```python
from build123d import *

# Parameters (mm, degrees)
HOLE_WIZARD_M31_AT_2_COUNT = 2
HOLE_WIZARD_M31_AT_2_PITCH = 12
HOLE_WIZARD_M31_AT_3_COUNT = 2
HOLE_WIZARD_M31_AT_3_PITCH = 8.485281374
HOLE_WIZARD_M31_AT_4_COUNT = 2
HOLE_WIZARD_M31_AT_4_PITCH = 8.485281374


with BuildPart() as part:
    # Эскиз1 → Повернуть1 (revolve)
    with BuildSketch(Plane(origin=(0, 0, 0), x_dir=(0, 0, -1), z_dir=(1, 0, 0))):
        with BuildLine():
            Line((-4, 9), (-3, 9))
            Line((-3, 9), (-3, 9.539392014))
            ThreePointArc((-3, 9.539392014), (0, 10), (3, 9.539392014))
            Line((3, 9.539392014), (3, 0))
            Line((3, 0), (-4, 0))
            Line((-4, 0), (-4, 9))
        make_face()
    revolve(axis=Axis((0, 0, 0), (0, 0, 1)))

    # Эскиз2 → Цековка для винта с внутренним шестигранником M31 (revolve, cut)
    with BuildSketch(Plane(origin=(6, 0, -3), x_dir=(0, 1, 0), z_dir=(1, 0, 0))):
        Polygon((0, 0), (0, 7), (1.9, 7), (1.7, 6.8), (1.7, 3.6), (1.9, 3.4), (3, 3.4), (3, 0.25), (3.25, 0), align=None)
    hole_wizard_m31 = revolve(axis=Axis((6, 0, -9.35), (0, 0, 1)), mode=Mode.SUBTRACT)

    # Цековка для винта с внутренним шестигранником M31 at 2: Цековка для винта с внутренним шестигранником M31 ×2
    with Locations(*[(-i * HOLE_WIZARD_M31_AT_2_PITCH, 0, 0) for i in range(1, HOLE_WIZARD_M31_AT_2_COUNT)]):
        add(hole_wizard_m31, mode=Mode.SUBTRACT)

    # Цековка для винта с внутренним шестигранником M31 at 3: Цековка для винта с внутренним шестигранником M31 ×2
    with Locations(*[Vector(-0.707106781, 0.707106781, 0) * (i * HOLE_WIZARD_M31_AT_3_PITCH) for i in range(1, HOLE_WIZARD_M31_AT_3_COUNT)]):
        add(hole_wizard_m31, mode=Mode.SUBTRACT)

    # Цековка для винта с внутренним шестигранником M31 at 4: Цековка для винта с внутренним шестигранником M31 ×2
    with Locations(*[Vector(-0.707106781, -0.707106781, 0) * (i * HOLE_WIZARD_M31_AT_4_PITCH) for i in range(1, HOLE_WIZARD_M31_AT_4_COUNT)]):
        add(hole_wizard_m31, mode=Mode.SUBTRACT)


solid = part.part
```
The listing builds one solid part. Answer for the finished solid, in the listing's coordinates (mm). A direction names the side the tool comes from. Round coordinates to 2 decimals unless told otherwise and drop trailing zeros. Write each loop counter-clockwise with the first axis right and the second up, starting at its lowest first coordinate (ties: lowest second). Pieces come first, ordered by that corner, then holes. Notation, with made-up numbers: (43.25, 83.25) -> (80.25, 83.25) arc R18 cw to (80.25, 114.25) -> close; hole circle Ø11 at (-5.5, 56.5). An arc over 180 degrees is marked (long way). Answer as a JSON object with one key per item and string values. Group by question number.
Q1. Section C-C (y = 0) is taken. Count the separate pieces of the cut face and the enclosed holes in it, plus the area to 3 significant figures.
Q2. Determine the mould class of faces 1 (the face through (0, 0, -3)), 2 (the face through (1.66, 5.63, 2.18)), 3 (the face through (-8.923, -1.172, 3.493)) for opening direction Y: pulls with the +Y half, pulls with the -Y half, needs draft (parallel to the pull), parting line crosses it, or undercut.
Q3. Straight lines are drawn through the part: line 1 along Y through (x, z) = (-0.5, 1); line 2 along X through (y, z) = (6, -1.2); line 3 along Z through (x, y) = (-4, 8.5). For each, find the intervals that lie inside material, in ascending order.
Q4. Each of these flat-tipped pins is pushed along its axis until it touches: pin 1 Ø3 at (x, y) = (6, 0) entering from +Z; pin 2 Ø1 at (x, z) = (5.5, -2) entering from +Y; pin 3 Ø3 at (x, y) = (5.5, 1.5) entering from -Z; pin 4 Ø3.5 at (x, y) = (0, 6) entering from -Z. Where does it stop, or does it pass through?
Q5. Which of the six approach directions +Z, -Z, +X, -X, +Y, -Y give full straight-line access (tool end or side, diameter ignored) to faces 4 (the face through (-5, -2, 0.4)), 5 (the face through (7.66, -0.37, 2.18)), 6 (the face through (7, 6, 3))?
Q6. Section A-A (x = -6) is taken. Write down the section's boundary in (y, z), plus the area to 3 significant figures.
Q7. Section D-D (z = 1.75) is taken. Write down the section's boundary in (x, y).
Check values:
{
 "1": {"separate pieces": "3", "enclosed holes": "0", "area": "70.6 mm^2"},
 "2": {"face 1": "needs draft", "face 2": "undercut", "face 3": "parting line crosses it"},
 "3": {"line 1": "-9.94 to -7.62, -4.38 to 4.38, 7.62 to 9.94", "line 2": "-7.91 to -3, 3 to 7.91", "line 3": "-3 to 3"},
 "4": {"pin 1": "through", "pin 2": "y = 8.45", "pin 3": "z = -2.83", "pin 4": "z = 0.55"},
 "5": {"face 4": "-Z", "face 5": "+Z, -Z", "face 6": "+Z"},
 "6": {"outline": "(-7.42, -3) -> (-3.25, -3) -> (-3, -2.75) -> (-3, 0.4) -> (-1.9, 0.4) -> (-1.7, 0.6) -> (-1.7, 3.8) -> (-1.9, 4) -> (-6.71, 4) -> (-6.71, 3) -> (-7.42, 3) arc R8 ccw to start; (1.7, 0.6) -> (1.9, 0.4) -> (3, 0.4) -> (3, -2.75) -> (3.25, -3) -> (7.42, -3) arc R8 ccw to (7.42, 3) -> (6.71, 3) -> (6.71, 4) -> (1.9, 4) -> (1.7, 3.8) -> close", "area": "74.3 mm^2"},
 "7": {"outline": "circle Ø19.69 at (0, 0); hole circle Ø3.4 at (-6, 0); hole circle Ø3.4 at (0, -6); hole circle Ø3.4 at (0, 6); hole circle Ø3.4 at (6, 0)"}
}
